from build123d import *

# Parameters (mm, degrees)
SKICA1_R                 = 3
P_IDAT_VYSUNUT_M1_DEPTH  = 23
SKICA2_R                 = 1.65
ODEBRAT_VYSUNUT_M1_DEPTH = 20
SKICA3_R                 = 3
P_IDAT_VYSUNUT_M2_DEPTH  = 5
SKICA4_R                 = 1.65
ODEBRAT_VYSUNUT_M2_DEPTH = 10


with BuildPart() as part:
    # Skica1 → Přidat vysunutím1 (new body)
    with BuildSketch(Plane.XY):
        Circle(SKICA1_R)
    extrude(amount=P_IDAT_VYSUNUT_M1_DEPTH)

    # Skica2 → Odebrat vysunutím1 (cut)
    with BuildSketch(Plane.XY.offset(23)):
        Circle(SKICA2_R)
    extrude(amount=-ODEBRAT_VYSUNUT_M1_DEPTH, mode=Mode.SUBTRACT)

    # Skica3 → Přidat vysunutím2 (add, symmetric)
    with BuildSketch(Plane(origin=(0, 0, 0), x_dir=(1, 0, 0), z_dir=(0, 1, 0))):
        with Locations((0, 2)):
            Circle(SKICA3_R)
    extrude(amount=P_IDAT_VYSUNUT_M2_DEPTH, both=True)

    # Skica4 → Odebrat vysunutím2 (cut)
    with BuildSketch(Plane(origin=(0, 5, 0), x_dir=(1, 0, 0), z_dir=(0, 1, 0))):
        with Locations((0, 1.995839667)):
            Circle(SKICA4_R)
    extrude(amount=-ODEBRAT_VYSUNUT_M2_DEPTH, mode=Mode.SUBTRACT)


solid = part.part
Design review of the part built by this model. Coordinates are the model's own, in mm. A direction names the side the tool comes from. Coordinates: 2 decimals unless noted, no trailing zeros. Loops run counter-clockwise (first coordinate to the right, second up) from the corner with the lowest first, then second, coordinate; pieces in that order, holes last. Notation, with made-up numbers: M -32,79.5 L 24,79.5 A27 ccw 24,111.5 Z; hole C 57,23 d2. An arc over 180 degrees is marked long. Answer as CSV lines item,"result".
Item 1: Machinability: for faces 4 (the face through (1.3, -5, -0.7)), 5 (the face through (-1.216, 1.115, 13.14)), which of the approach directions +Z, -Z, +X, -X, +Y, -Y give a long, thin tool a straight path to every point of the face, cutting with its end or side? Answer none if there is none.
Answer list:
face 4,"+Z, -Z, +X, -X, -Y"
face 5,"+Z"
Item 2: Add section A-A on x = 0. State the section outline as (y, z) points, plus the area to 3 significant figures.
Answer list:
outline,"M -5,-5 L 5,-5 L 5,-3.65 L -5,-3.65 Z; M -5,-0.35 L 5,-0.35 L 5,1 L 3,1 L 3,23 L 1.65,23 L 1.65,3 L -1.65,3 L -1.65,23 L -3,23 L -3,1 L -5,1 Z"
area,"93.0 mm²"
Item 3: For P1, Ø0.8, axis at x = 2.5, y = 0.5, coming from the -Z side; P2, Ø1, axis at x = -2, z = 13.5, coming from the +Y side; P3, Ø1.5, axis at x = 1.5, z = 18.5, coming from the +Y side, all flat-tipped, find the tip position at first contact; note any pin that passes through.
Answer list:
P1,"z = -4.14"
P2,"y = 2.6"
P3,"y = 2.9"
Item 4: The part is to be moulded in two halves that separate along X. For faces 1 (the face through (0, 0, 3)), 2 (the face through (1.3, -1.3, 23)), 3 (the face through (-3, 0, 11)), say which applies: pulls with the +X half, pulls with the -X half, needs draft (parallel to the pull), parting line crosses it, or undercut.
Answer list:
face 1,"undercut"
face 2,"needs draft"
face 3,"parting line crosses it"
Item 5: For probe 1 along Y at (x, z) = (0, 7.75); probe 2 along Z at (x, y) = (0, -1), list the stretches that pass through material, from the lowest coordinate up.
Answer list:
probe 1,"-3 to -1.65, 1.65 to 3"
probe 2,"-5 to -3.65, -0.35 to 3"
Item 6: Add section C-C on z = 5.5. State the section outline as (x, y) points.
Answer list:
outline,"C 0,0 d6; hole C 0,0 d3.3"
Item 7: Add section B-B on y = 0.5. State the section outline as (x, z) points.
Answer list:
outline,"M -2.96,0 L -2.24,0 A3 ccw long 2.24,0 L 2.96,0 L 2.96,23 L 1.57,23 L 1.57,3 L -1.57,3 L -1.57,23 L -2.96,23 Z; hole C 0,-2 d3.3"
Item 8: Add section D-D on y = -2.25. State the section outline as (x, z) points, plus the area to 3 significant figures.
Answer list:
outline,"M -1.98,0.25 A3 ccw long 1.98,0.25 L 1.98,23 L -1.98,23 Z; hole C 0,-2 d3.3"
area,"108 mm²"
